Autodesk Inventor part; units mm, degrees
ref_plane "YZ Plane" through (0, 0, 0) normal (1, 0, 0) x (0, 1, 0)
ref_plane "XZ Plane" through (0, 0, 0) normal (0, 1, 0) x (-1, 0, 0)
ref_plane "XY Plane" through (0, 0, 0) normal (0, 0, 1) x (1, 0, 0)
sketch "Sketch1" plane through (0, 0, 0) normal (0, 1, 0) x (-1, 0, 0)
  line L0 (0, 0) -> (28.575, 0)
  line L1 (28.575, 0) -> (0, 0)
  line L2 (0, 0) -> (-14.2875, -24.7467)
  line L3 (0, 0) -> (28.575, 0) construction
  line L4 (0, 0) -> (-14.2875, 24.7467)
  line L5 (0, 0) -> (28.575, 0) construction
  circle A0 centre (28.575, 0) radius 2.54
  circle A1 centre (-14.2875, -24.7467) radius 2.54
  circle A2 centre (-14.2875, 24.7467) radius 2.54
  circle A3 centre (0, 0) radius 3.175
  circle A4 centre (0, 0) radius 6.35
  line L6 (-1.5875, -2.7496) -> (0, 0)
  line L7 (0, 0) -> (-6.35, 0)
  circle A5 centre (-14.2875, 24.7467) radius 3.81
  circle A6 centre (28.575, 0) radius 3.81
  circle A7 centre (-14.2875, -24.7467) radius 3.81
  line L8 (30.6811, 3.175) -> (-12.1814, 27.9217)
  line L9 (28.2054, -3.792) -> (-10.8187, -26.3226)
  line L10 (-18.0975, 24.7467) -> (-18.0975, -24.7467)
  line L11 (0, 0) -> (5.0525, -8.8146)
  line L12 (0, 0) -> (5.1463, 8.7602)
  line L13 (0, 0) -> (-10.16, 0)
  arc A8 (28.2054, -3.792) -> (-10.8187, -26.3226) centre (24.4473, -42.344) ccw
  arc A9 (-10.8187, 26.3226) -> (28.2054, 3.792) centre (24.4473, 42.344) ccw
  arc A10 (-17.3867, -22.5305) -> (-17.3867, 22.5305) centre (-48.8947, 0) ccw
  point P0 (5.1074, 8.7829)
  point P1 (-10.16, 0.0317)
  point P2 (30.2716, 3.4114)
  point P3 (28.2054, 3.792)
  point P4 (-10.8187, 26.3226)
  point P5 (-17.3867, 22.5305)
  point P6 (-17.3867, -22.5305)
  dimension "d9" = 6.35
  dimension "d41" = 12.7
  dimension "d0" = 28.575
  dimension "d1" = 28.575
  dimension "d2" = 120
  dimension "d3" = 28.575
  dimension "d4" = 120
  dimension "d5" = 5.08
  dimension "d6" = 5.08
  dimension "d7" = 5.08
  dimension "d42" = 7.62
  dimension "d43" = 7.62
  dimension "d44" = 7.62
  dimension "d47" = 10.16
  dimension "d48" = 10.16
  dimension "d49" = 10.16
  dimension "d52" = 360
extrude "Extrusion4" add sketch "Sketch1" along normal blind 12.7 contours A3 L12 A4 L0 | L0 A4 L11 A3 | A3 L11 A4 L2 | L2 A4 L7 A3 | A3 L7 A4 L4 | L4 A4 L12 A3 | A4 L12 A9 A6 L0 | L0 A6 A8 L11 A4 | A4 L11 A8 A7 L2 | L2 A7 A10 L13 A4 | A4 L13 A10 A5 L4 | L4 A5 A9 L12 A4 | A6 L8 | A7 | A5 picked at (31.8987, 0.5122)
sketch "Sketch15" plane through (0, 12.7, 0) normal (0, 1, 0) x (1, 0, 0)
  circle A0 centre (-28.575, 0) radius 2.54
  line L0 (-28.575, 0) -> (-10.541, 0)
  circle A1 centre (14.2875, 24.7467) radius 2.54
  circle A2 centre (14.2875, -24.7467) radius 2.54
  line L1 (14.2875, -24.7467) -> (5.2705, -9.1288)
  line L2 (14.2875, 24.7467) -> (5.2705, 9.1288)
  line L3 (-10.541, 0) -> (-10.541, 6.1917)
  arc A3 (-28.2054, 3.792) -> (10.8187, 26.3226) centre (-24.4473, 42.344) ccw
  line L4 (-10.541, 0) -> (-10.541, -6.1917)
  arc A4 (10.8187, -26.3226) -> (-28.2054, -3.792) centre (-24.4473, -42.344) ccw
  arc A5 (17.3867, 22.5305) -> (17.3867, -22.5305) centre (48.8947, 0) ccw
  line L5 (5.2705, -9.1288) -> (10.6326, -6.0329)
  line L6 (5.2705, -9.1288) -> (-0.0916, -12.2246)
  line L7 (5.2705, 9.1288) -> (-0.0916, 12.2246)
  line L8 (5.2705, 9.1288) -> (10.6326, 6.0329)
  arc A6 (10.8187, -26.3226) -> (17.3867, -22.5305) centre (14.2875, -24.7467) ccw
  arc A7 (17.3867, 22.5305) -> (10.8187, 26.3226) centre (14.2875, 24.7467) ccw
  arc A8 (-28.2054, 3.792) -> (-30.6811, -3.175) centre (-28.575, 0) ccw
  line L9 (-30.6811, -3.175) -> (-30.2716, -3.4114)
  arc A9 (-30.2716, -3.4114) -> (-28.2054, -3.792) centre (-28.575, 0) ccw
  point P0 (0, 0)
  dimension "d91" = 18.034
  dimension "d92" = 18.034
  dimension "d93" = 18.034
extrude "Extrusion7" cut sketch "Sketch15" against normal blind 25.4 contours L4 A4 A9 L9 A8 A3 L3 | A3 A7 A5 L8 L7 | L6 L5 A5 A6 A4
sketch "Sketch16" plane through (10.6326, 0, 6.0329) normal (0.5, 0, 0.8660254) x (0.8660254, 0, -0.5)
  line L0 (-9.3667, 12.7) -> (-3.0167, 12.7)
  line L1 (-6.1917, 12.7) -> (-6.1917, 0)
  line L2 (-12.3833, 0) -> (-12.3833, 12.7)
  line L3 (-12.3833, 6.35) -> (0, 6.35)
  line L4 (0, 12.7) -> (0, 0)
  circle A0 centre (-6.1917, 6.35) radius 1.27
  dimension "d96" = 2.54
extrude "Extrusion8" cut sketch "Sketch16" against normal blind 6.35
thread "Thread1"
pattern_circular "Circular Pattern1" count 3 over 360 about axis through (0, 0, 0) along (0, 1, 0) of "Extrusion8"
properties part number "stability copy"
Design review of the part built by this model. Coordinates are the model's own, in mm. A direction names the side the tool comes from. Give positions to 0.01 mm unless a question says otherwise; leave off trailing zeros. Write each loop counter-clockwise with the first axis right and the second up, starting at its lowest first coordinate (ties: lowest second). Pieces come first, ordered by that corner, then holes. Notation, with made-up numbers: M 42,-3.75 L 56,-3.75 A14 ccw 56,23.25 Z; hole C 8.5,49 d7. An arc over 180 degrees is marked long. Answer as a JSON object with one key per item and string values. Group by question number.
1) We need section B-B (y = 6.35). Give the boundary of the cut face in (x, z) (3 decimals), and give its area (3 significant figures).
2) We need section A-A (x = -0.75). Give the boundary of the cut face in (y, z).
3) For line 1 along Z through (x, y) = (4.25, 7); line 2 along X through (y, z) = (5.75, -0.75); line 3 along X through (y, z) = (6.5, 6), list the stretches that pass through material, from the lowest coordinate up.
4) Clearance check with flat-ended pins moving along their axes: pin 1 Ø5 at (y, z) = (8.5, 5.5) entering from +X; pin 2 Ø2 at (y, z) = (6.35, 0) entering from -X; pin 3 Ø1 at (x, y) = (-6.5, 2) entering from +Z. State where each tip first meets the part, or that it passes through.
5) Tool access review of faces 1 (the face through (2.079, 6.368, 3.637)), 2 (the face through (-4.189, 6, 0)): name each direction out of +Z, -Z, +X, -X, +Y, -Y from which nothing blocks a thin tool from reaching the whole face with its end or side.
6) Mouldability with a two-part tool opening along Y and no side actions: class faces 3 (the face through (3.85, 7.61, -6.33)), 4 (the face through (-10.541, 6.4, -1.5)) as released by +Y, released by -Y, zero draft, split by the parting line, or undercut.
Answer key:
{
 "1": {"outline": "M -10.541,-6.192 A38.735 cw -0.092,-12.225 L 4.171,-9.764 L 0.995,-4.263 L 3.194,-2.993 L 6.37,-8.494 L 10.633,-6.033 A38.735 cw 10.633,6.033 L 6.37,8.494 L 3.194,2.993 L 0.995,4.263 L 4.171,9.764 L -0.092,12.225 A38.735 cw -10.541,6.192 L -10.541,1.27 L -4.189,1.27 L -4.189,-1.27 L -10.541,-1.27 Z; hole C 0,0 d6.35", "area": "297 mm²"},
 "2": {"outline": "M 0,-11.7 L 12.7,-11.7 L 12.7,-3.09 L 0,-3.09 Z; M 0,3.09 L 12.7,3.09 L 12.7,11.7 L 0,11.7 Z"},
 "3": {"line 1": "z = -9.72 to -9.54, -5.18 to 5.18, 9.54 to 9.72", "line 2": "x = -4.19 to -3.09, 3.09 to 10.17", "line 3": "x = -10.54 to 2.01, 4.92 to 10.63"},
 "4": {"pin 1": "stops at x = 10.63", "pin 2": "stops at x = -4.19", "pin 3": "stops at z = 8.28"},
 "5": {"face 1": "none", "face 2": "-X"},
 "6": {"face 3": "undercut", "face 4": "zero draft"}
}
